Input: part model. Units: mm. Frame: model coordinates. Face numbers are marked on the shaded views. A direction names the side the tool comes from. Round coordinates to 2 decimals unless told otherwise and drop trailing zeros. Write each loop counter-clockwise with the first axis right and the second up, starting at its lowest first coordinate (ties: lowest second). Pieces come first, ordered by that corner, then holes. Notation, with made-up numbers: (18.25, 57.25) -> (32.25, 57.25) arc R24 cw to (32.25, 82.25) -> close; hole circle Ø3 at (47, -20.75). An arc over 180 degrees is marked (long way). Use CSV: the item, a comma, the result in double quotes.
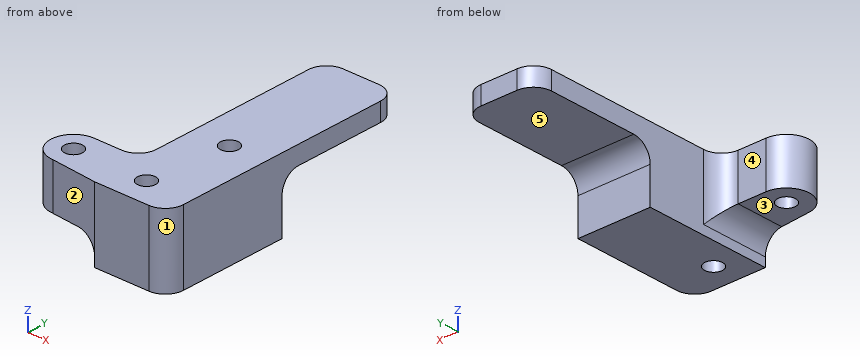
Autodesk Inventor part; units mm, degrees
ref_plane "YZ Plane" through (0, 0, 0) normal (1, 0, 0) x (0, 1, 0)
ref_plane "XZ Plane" through (0, 0, 0) normal (0, 1, 0) x (-1, 0, 0)
ref_plane "XY Plane" through (0, 0, 0) normal (0, 0, 1) x (1, 0, 0)
sketch "Sketch1" plane through (0, 0, 0) normal (0, 0, 1) x (1, 0, 0)
  circle A0 centre (30, 0) radius 1
  circle A1 centre (21.926, 0) radius 1
  line L0 (27, 11) -> (35, 11)
  line L1 (35, 11) -> (35, -3)
  line L2 (35, -3) -> (27, -3)
  line L3 (27, -3) -> (27, 11)
  circle A2 centre (21.926, 0) radius 2.5
  line L4 (21.926, -2.5) -> (27, -3)
  line L5 (21.926, 2.5) -> (27, 2.5)
  point P0 (0, 0)
  dimension "d0" = 21.926
  dimension "d1" = 30
  dimension "d2" = 2
  dimension "d3" = 2
  dimension "d4" = 3
  dimension "d5" = 5
  dimension "d6" = 3
  dimension "d7" = 11
  dimension "d8" = 5
extrude "Extrusion1" add sketch "Sketch1" along normal blind 8
fillet "Fillet1" radius 2 2 edges at (27, 2.5, 4) (35, -3, 4)
sketch "Sketch2" plane through (0, 0, 8) normal (0, 0, 1) x (1, 0, 0)
  line L0 (27, 11) -> (27, 4.5)
  line L1 (27, 11) -> (35, 11)
  line L2 (35, 11) -> (35, 25)
  line L3 (35, 25) -> (27, 25)
  line L4 (27, 25) -> (27, 11)
  line L5 (35, -1) -> (35, 11)
  circle A0 centre (30, 0) radius 1
  point P0 (0, 0)
  dimension "d12" = 25
extrude "Extrusion2" add sketch "Sketch2" against normal blind 2 contours L4 L3 L2 L1
fillet "Fillet2" radius 2 1 edges at (31, 11, 6)
fillet "Fillet3" radius 2 2 edges at (35, 25, 7) (27, 25, 7)
sketch "Sketch3" plane through (0, 0, 8) normal (0, 0, 1) x (1, 0, 0)
  line L0 (35, -1) -> (35, 23)
  line L1 (27, 23) -> (27, 4.5)
  circle A0 centre (30, 0) radius 1
  point P0 (0, 0)
  point P1 (31, 9)
  dimension "d17" = 8
  dimension "d18" = 4
  dimension "d19" = 9
hole "Hole1" at (31, 9, 8) direction (0, 0, -1) diameter 2 depth 5 tip angle 118
sketch "Sketch4" plane through (0, 0, 0) normal (0, 0, -1) x (-1, 0, 0)
  line L0 (-27, 11) -> (-27, 4.5)
  line L1 (-17, -3) -> (-27, -3)
  line L2 (-27, -3) -> (-27, 5)
  line L3 (-27, 5) -> (-17, 5)
  line L4 (-17, 5) -> (-17, -3)
  line L5 (-27, -3) -> (-33, -3)
  point P0 (0, 0)
  dimension "d27" = 10
  dimension "d28" = 8
extrude "Extrusion3" cut sketch "Sketch4" against normal blind 3
fillet "Fillet4" radius 2 1 edges at (27, 0.75, 3)
properties part number "front_v2"
Item 1: Set-up query: the marked faces 1, 2, 3, 4 and 5. Return all of +Z, -Z, +X, -X, +Y, -Y with unobstructed straight access to the full face (end or side cutting, diameter ignored); none if empty.
Worked answers:
face 1,"+Z, -Z, +X, -Y"
face 2,"+Z, -Z, -X, -Y"
face 3,"-Z, -X, +Y, -Y"
face 4,"+Z, -Z, -X, +Y"
face 5,"-Z, +X, -X, +Y"
Item 2: Line query: line 1 (Y direction, x = 30.25, z = 6.5); line 2 (X direction, y = 9, z = 4.75); line 3 (X direction, y = 10.5, z = 4.25). Output: solid intervals per line, ascending.
Worked answers:
line 1,"y = -3 to -0.97, 0.97 to 8.34, 9.66 to 25"
line 2,"x = 27 to 30, 32 to 35"
line 3,"x = 27 to 35"
Item 3: Section query C-C on x = 28.5. Return the cut outline in (y, z).
Worked answers:
outline,"(-3, 0) -> (11, 0) -> (11, 4) arc R2 cw to (13, 6) -> (24.94, 6) -> (24.94, 8) -> (-3, 8) -> close"
Item 4: First-contact query: pin 1 Ø6.5 at (x, y) = (32, 20) entering from -Z; pin 2 Ø3 at (x, y) = (24.5, 21) entering from +Z; pin 3 Ø4.5 at (x, z) = (32, 1) entering from +Y; pin 4 Ø4 at (x, y) = (21, -0.5) entering from -Z. Flat tips, straight axial feed; report the tip coordinate or a pass-through.
Worked answers:
pin 1,"stops at z = 6"
pin 2,"passes through"
pin 3,"stops at y = 11"
pin 4,"stops at z = 3"
Item 5: Section query B-B on z = 7.25. Return the cut outline in (x, y), plus the area to 3 significant figures.
Worked answers:
outline,"(21.93, -2.5) -> (27, -3) -> (33, -3) arc R2 ccw to (35, -1) -> (35, 23) arc R2 ccw to (33, 25) -> (29, 25) arc R2 ccw to (27, 23) -> (27, 4.5) arc R2 cw to (25, 2.5) -> (21.93, 2.5) arc R2.5 ccw to start; hole circle Ø2 at (21.93, 0); hole circle Ø2 at (30, 0); hole circle Ø2 at (31, 9)"
area,"249 mm²"
Item 6: Section query D-D on z = 0.5. Return the cut outline in (x, y).
Worked answers:
outline,"(27, -3) -> (33, -3) arc R2 ccw to (35, -1) -> (35, 11) -> (27, 11) -> close; hole circle Ø2 at (30, 0)"
Item 7: Section query A-A on y = 0. Return the cut outline in (x, z).
Worked answers:
outline,"(19.43, 3) -> (20.93, 3) -> (20.93, 8) -> (19.43, 8) -> close; (22.93, 3) -> (25, 3) arc R2 cw to (27, 1) -> (27, 0) -> (29, 0) -> (29, 8) -> (22.93, 8) -> close; (31, 0) -> (35, 0) -> (35, 8) -> (31, 8) -> close"
